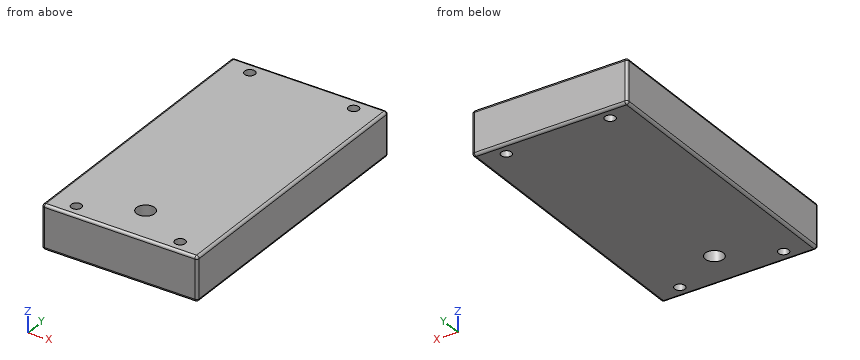
```python
from build123d import *

# Parameters (mm, degrees)
F0_W     = 60
F0_H     = 110
F0_R     = 2
F1_DEPTH = 8.5
F2_R     = 1
F3_R     = 3.5
F4_DEPTH = 25


with BuildPart() as f1:
    # F0 (on Top) → F1 (new body, symmetric)
    with BuildSketch(Plane.XY):
        Rectangle(F0_W, F0_H)
        with Locations((-20, -50)):
            Circle(F0_R, mode=Mode.SUBTRACT)
        with Locations((20, -50)):
            Circle(F0_R, mode=Mode.SUBTRACT)
        with Locations((-20, 50)):
            Circle(F0_R, mode=Mode.SUBTRACT)
        with Locations((20, 50)):
            Circle(F0_R, mode=Mode.SUBTRACT)
    extrude(amount=F1_DEPTH, both=True)

    # F2
    f2_edges = [f1.edges().sort_by_distance(p)[0] for p in [
        (30, 0, 8.5),
        (0, -55, 8.5),
        (-30, 0, 8.5),
        (0, 55, 8.5),
        (30, 0, -8.5),
        (30, -55, 0),
        (30, 55, 0),
        (0, 55, -8.5),
        (-30, 0, -8.5),
        (-30, 55, 0),
        (-30, -55, 0),
        (0, -55, -8.5),
    ]]
    fillet(f2_edges, radius=F2_R)

    # F3 (on face) → F4 (cut)
    with BuildSketch(Plane.XY.offset(8.5)):
        with Locations((0, -40)):
            Circle(F3_R)
    extrude(amount=-F4_DEPTH, mode=Mode.SUBTRACT)


solid = f1.part
```
Build history of the part. All positions in model axes, mm. Round coordinates to 2 decimals unless told otherwise and drop trailing zeros. Loops run counter-clockwise (first coordinate to the right, second up) from the corner with the lowest first, then second, coordinate; pieces in that order, holes last.
Item 1: Saw through at A-A (y = -50). List the corners of the cut face in (x, z), then the cut area to 3 significant figures.
Item 2: Drill centre lines: line 1 along Y through (x, z) = (-20, -4.5); line 2 along Y through (x, z) = (21.5, -3); line 3 along Y through (x, z) = (0, -4). Where is each one in solid material? Low to high.
Item 3: Saw through at B-B (x = 20). List the corners of the cut face in (y, z), then the cut area to 3 significant figures.
Worked answers:
1. outline: (-30, -7.5) arc R1 ccw to (-29, -8.5) - (-22, -8.5) - (-22, 8.5) - (-29, 8.5) arc R1 ccw to (-30, 7.5) - close; (-18, -8.5) - (18, -8.5) - (18, 8.5) - (-18, 8.5) - close; (22, -8.5) - (29, -8.5) arc R1 ccw to (30, -7.5) - (30, 7.5) arc R1 ccw to (29, 8.5) - (22, 8.5) - close
1. area: 883 mm2
2. line 1: y = -55 to -52, -48 to 48, 52 to 55
2. line 2: y = -55 to -51.32, -48.68 to 48.68, 51.32 to 55
2. line 3: y = -55 to -43.5, -36.5 to 55
3. outline: (-55, -7.5) arc R1 ccw to (-54, -8.5) - (-52, -8.5) - (-52, 8.5) - (-54, 8.5) arc R1 ccw to (-55, 7.5) - close; (-48, -8.5) - (48, -8.5) - (48, 8.5) - (-48, 8.5) - close; (52, -8.5) - (54, -8.5) arc R1 ccw to (55, -7.5) - (55, 7.5) arc R1 ccw to (54, 8.5) - (52, 8.5) - close
3. area: 1,730 mm2
